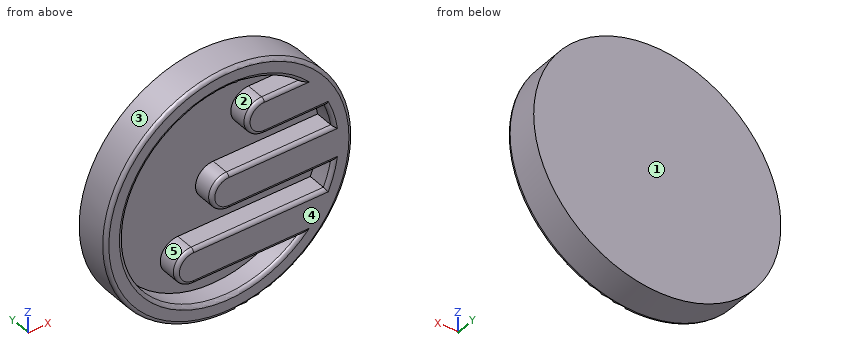
from build123d import *

# Parameters (mm, degrees)
F0_R     = 44.45
F1_DEPTH = 12.7
F2_R     = 44.45
F3_DEPTH = 5.08
F4_R     = 1.27


with BuildPart() as f1:
    # F0 (on Front) → F1 (new body)
    with BuildSketch(Plane.XZ):
        Circle(F0_R)
        with BuildLine():
            ThreePointArc((25.903019, -27.94), (-38.1, 0), (25.903019, 27.94))
            Line((25.903019, 27.94), (12.7, 27.94))
            ThreePointArc((12.7, 27.94), (6.35, 21.59), (12.7, 15.24))
            Line((12.7, 15.24), (34.919227, 15.24))
            ThreePointArc((34.919227, 15.24), (36.514725, 10.875883), (37.567107, 6.35))
            Line((37.567107, 6.35), (0, 6.35))
            ThreePointArc((0, 6.35), (-6.35, 0), (0, -6.35))
            Line((0, -6.35), (37.567107, -6.35))
            ThreePointArc((37.567107, -6.35), (36.514725, -10.875883), (34.919227, -15.24))
            Line((34.919227, -15.24), (0, -15.24))
            Line((0, -15.24), (-12.7, -15.24))
            ThreePointArc((-12.7, -15.24), (-19.05, -21.59), (-12.7, -27.94))
            Line((-12.7, -27.94), (0, -27.94))
            Line((0, -27.94), (25.903019, -27.94))
        make_face(mode=Mode.SUBTRACT)
    extrude(amount=F1_DEPTH)

    # F2 (on Front) → F3 (join)
    with BuildSketch(Plane.XZ):
        Circle(F2_R)
    extrude(amount=F3_DEPTH)

    # F4
    f4_edges = [f1.edges().sort_by_distance(p)[0] for p in [
        (-44.45, -12.7, 0),
        (6.60151, -12.7, -27.94),
        (18.783553, -12.7, -6.35),
        (23.809613, -12.7, 15.24),
        (36.514725, -12.7, -10.875883),
        (36.514725, -12.7, 10.875883),
        (-38.1, -12.7, 0),
    ]]
    fillet(f4_edges, radius=F4_R)


solid = f1.part
Can you work these out from the model? Positions are in its coordinate system, mm. Face numbers are marked on the shaded views. A direction names the side the tool comes from. Coordinates: 2 decimals unless noted, no trailing zeros. Order: outer loops, then holes, each group sorted by start corner. A loop starts at its lowest first (then second) coordinate and runs counter-clockwise, first axis right, second up. Notation, with made-up numbers: (-6, 83.25) - (24, 83.25) arc R25 ccw to (24, 100.25) - close; hole circle Ø11 at (12.25, 32). An arc over 180 degrees is marked (long way). Answer as a JSON object with one key per item and string values. Group by question number.
Q1. Will these pins go through, and if not, where does the flat tip stop? P1, Ø1.9, axis at x = 13.5, y = -9.5, coming from the -Z side; P2, Ø2, axis at x = 15, y = -8.5, coming from the +Z side; P3, Ø22.5, axis at x = -6, z = 18.5, coming from the -Y side.
Q2. Imagine slicing it at B-B (y = -7.75). Please give me the cut outline in (x, z).
Q3. Imagine slicing it at A-A (z = 0). Please give me the cut outline in (x, y), and give its area (3 significant figures).
Q4. We'd pull the mould along Z, two halves only. Please class the marked faces 1, 2 and 3: +Z half, -Z half, draft (parallel to the pull), parting line (faces both ways), or undercut.
Q5. On a 3-axis mill with a long thin cutter (end or side, diameter ignored), from which of +Z, -Z, +X, -X, +Y, -Y can I reach the whole of each face in a straight line? I mean the marked faces 4 and 5. Say none if no direction works.
Q6. I need wall thicknesses on line 1 (Z direction, x = 0, y = -9.75); line 2 (Z direction, x = -17, y = -10.5). Which ranges of each line are inside material? Lowest first, please. Write a range as from..to.
Determined:
{
 "1": {"P1": "stops at z = -42.64", "P2": "stops at z = 42.19", "P3": "stops at y = -5.08"},
 "2": {"outline": "circle Ø88.9 at (0, 0); hole (-12.7, -27.94) arc R6.35 cw to (-12.7, -15.24) - (34.92, -15.24) arc R38.1 ccw to (37.57, -6.35) - (0, -6.35) arc R6.35 cw to (0, 6.35) - (37.57, 6.35) arc R38.1 ccw to (34.92, 15.24) - (12.7, 15.24) arc R6.35 cw to (12.7, 27.94) - (25.9, 27.94) arc R38.1 ccw (long way) to (25.9, -27.94) - close"},
 "3": {"outline": "(-44.45, -11.43) arc R1.27 ccw to (-43.18, -12.7) - (-39.37, -12.7) arc R1.27 ccw to (-38.1, -11.43) - (-38.1, -5.08) - (-6.35, -5.08) - (-6.35, -11.43) arc R1.27 ccw to (-5.08, -12.7) - (43.18, -12.7) arc R1.27 ccw to (44.45, -11.43) - (44.45, 0) - (-44.45, 0) - close", "area": "886 mm2"},
 "4": {"face 1": "draft", "face 2": "undercut", "face 3": "parting line"},
 "5": {"face 4": "+Z, -Z, +X, -X, -Y", "face 5": "-Y"},
 "6": {"line 1": "z = -44.45..-38.1, -27.94..-15.24, -6.35..6.35, 38.1..44.45", "line 2": "z = -41.07..-34.1, -26.26..-16.92, 34.1..41.07"}
}
